```python
from build123d import *

# Parameters (mm, degrees)
SKETCH1_R           = 23.241
BOSS_EXTRUDE1_DEPTH = 38.1
CUT_EXTRUDE1_REACH  = 40.1
SKETCH2_R           = 3.302
CUT_EXTRUDE2_REACH  = 40.1
SKETCH3_R           = 3.302


with BuildPart() as part:
    # Sketch1 → Boss-Extrude1 (new body)
    with BuildSketch(Plane(origin=(0, 0, 0), x_dir=(1, 0, 0), z_dir=(0, 1, 0))):
        Circle(SKETCH1_R)
    extrude(amount=BOSS_EXTRUDE1_DEPTH)

    # Sketch2 → Cut-Extrude1 (cut, up to next)
    with BuildSketch(Plane(origin=(0, 38.1, 0), x_dir=(1, 0, 0), z_dir=(0, 1, 0)), mode=Mode.PRIVATE) as cut_extrude1_sk1:
        with Locations((19.685, 0)):
            Circle(SKETCH2_R)
    cut_extrude1_tool1 = extrude(cut_extrude1_sk1.sketch, amount=-CUT_EXTRUDE1_REACH, mode=Mode.PRIVATE) & part.part
    add(cut_extrude1_tool1.solids().sort_by_distance((19.685, 38.1, 0))[0], mode=Mode.SUBTRACT)
    # Sketch2 → Cut-Extrude1 (cut, up to next)
    with BuildSketch(Plane(origin=(0, 38.1, 0), x_dir=(1, 0, 0), z_dir=(0, 1, 0)), mode=Mode.PRIVATE) as cut_extrude1_sk2:
        with Locations((-19.685, 0)):
            Circle(SKETCH2_R)
    cut_extrude1_tool2 = extrude(cut_extrude1_sk2.sketch, amount=-CUT_EXTRUDE1_REACH, mode=Mode.PRIVATE) & part.part
    add(cut_extrude1_tool2.solids().sort_by_distance((-19.685, 38.1, 0))[0], mode=Mode.SUBTRACT)

    # Sketch3 → Cut-Extrude2 (cut, up to next)
    with BuildSketch(Plane(origin=(0, 38.1, 0), x_dir=(1, 0, 0), z_dir=(0, 1, 0)), mode=Mode.PRIVATE) as cut_extrude2_sk1:
        Circle(SKETCH3_R)
    cut_extrude2_tool1 = extrude(cut_extrude2_sk1.sketch, amount=-CUT_EXTRUDE2_REACH, mode=Mode.PRIVATE) & part.part
    add(cut_extrude2_tool1.solids().sort_by_distance((0, 38.1, 0))[0], mode=Mode.SUBTRACT)


solid = part.part
```
Verification items for the finished model (mm, model axes). Coordinates: 2 decimals unless noted, no trailing zeros. Loops run counter-clockwise (first coordinate to the right, second up) from the corner with the lowest first, then second, coordinate; pieces in that order, holes last. Notation, with made-up numbers: (-12.5, 28.25) -> (1.5, 28.25) arc R20 cw to (1.5, 35.25) -> close; hole circle Ø6 at (49.25, -29). An arc over 180 degrees is marked (long way). Put each result on its own line as item: value.
1. Section check D-D, the plane z = 16. Record the boundary of the cut face in (x, y), then the cut area to 3 significant figures.
Result set:
outline: (-16.86, 0) -> (16.86, 0) -> (16.86, 38.1) -> (-16.86, 38.1) -> close
area: 1,280 mm^2
2. Section check B-B, the plane z = 0. Record the boundary of the cut face in (x, y).
Result set:
outline: (-23.24, 0) -> (-22.99, 0) -> (-22.99, 38.1) -> (-23.24, 38.1) -> close; (-16.38, 0) -> (-3.3, 0) -> (-3.3, 38.1) -> (-16.38, 38.1) -> close; (3.3, 0) -> (16.38, 0) -> (16.38, 38.1) -> (3.3, 38.1) -> close; (22.99, 0) -> (23.24, 0) -> (23.24, 38.1) -> (22.99, 38.1) -> close
3. Section check C-C, the plane y = 36. Record the boundary of the cut face in (x, z) (3 decimals).
Result set:
outline: circle Ø46.482 at (0, 0); hole circle Ø6.604 at (-19.685, 0); hole circle Ø6.604 at (0, 0); hole circle Ø6.604 at (19.685, 0)
4. Gauge pin test, flat ends, axial feed: P1, Ø2, axis at y = 26, z = 8.5, coming from the -X side; P2, Ø12, axis at x = 5, y = 23, coming from the -Z side; P3, Ø1.5, axis at x = 14, y = 22.5, coming from the -Z side. Record the tip position at first contact, or that the pin passes through.
Result set:
P1: stops at x = -22
P2: stops at z = -23.24
P3: stops at z = -19.09
5. Mould release check, pull along Z, two halves, no side actions. Record for faces 1 (the face through (0, 0, 5)), 2 (the face through (16.386, 19.317, -0.145)), 3 (the face through (3.05, 19.32, 1.26)), 4 (the face through (10.72, 18.78, 20.62)): pulls with the +Z half, pulls with the -Z half, needs draft (parallel to the pull), parting line crosses it, or undercut.
Result set:
face 1: needs draft
face 2: undercut
face 3: undercut
face 4: parting line crosses it
6. Thickness scan on line 1 (X direction, y = 14, z = 0); line 2 (Z direction, x = 0, y = 13.5); line 3 (X direction, y = 31, z = -2.5). Record the ranges inside material, lowest first.
Result set:
line 1: x = -23.24 to -22.99, -16.38 to -3.3, 3.3 to 16.38, 22.99 to 23.24
line 2: z = -23.24 to -3.3, 3.3 to 23.24
line 3: x = -23.11 to -21.84, -17.53 to -2.16, 2.16 to 17.53, 21.84 to 23.11
7. Section check A-A, the plane x = 0. Record the boundary of the cut face in (y, z).
Result set:
outline: (0, -23.24) -> (38.1, -23.24) -> (38.1, -3.3) -> (0, -3.3) -> close; (0, 3.3) -> (38.1, 3.3) -> (38.1, 23.24) -> (0, 23.24) -> close
